from build123d import *

# Parameters (mm, degrees)
SKETCH1_W           = 127
SKETCH1_H           = 508
BOSS_EXTRUDE1_DEPTH = 95.25
SKETCH2_W           = 88.9
SKETCH2_H           = 469.9
CUT_EXTRUDE2_DEPTH  = 88.9
CUT_EXTRUDE3_DEPTH  = 128
SKETCH4_W           = 127
SKETCH4_H           = 19.05
CUT_EXTRUDE4_DEPTH  = 50.8


with BuildPart() as part:
    # Sketch1 → Boss-Extrude1 (new body)
    with BuildSketch(Plane(origin=(0, 0, 0), x_dir=(1, 0, 0), z_dir=(0, 1, 0))):
        Rectangle(SKETCH1_W, SKETCH1_H)
    extrude(amount=BOSS_EXTRUDE1_DEPTH)

    # Sketch2 → Cut-Extrude2 (cut)
    with BuildSketch(Plane(origin=(0, 95.25, 0), x_dir=(1, 0, 0), z_dir=(0, 1, 0))):
        Rectangle(SKETCH2_W, SKETCH2_H)
    extrude(amount=-CUT_EXTRUDE2_DEPTH, mode=Mode.SUBTRACT)

    # Sketch3 → Cut-Extrude3 (cut, through all)
    with BuildSketch(Plane(origin=(63.5, 0, 0), x_dir=(0, 0, -1), z_dir=(1, 0, 0))):
        with BuildLine():
            Line((203.2, 38.1), (-215.9, 38.1))
            ThreePointArc((-215.9, 38.1), (-228.6, 50.8), (-215.9, 63.5))
            Line((-215.9, 63.5), (203.2, 63.5))
            ThreePointArc((203.2, 63.5), (215.9, 50.8), (203.2, 38.1))
        make_face()
    extrude(amount=-CUT_EXTRUDE3_DEPTH, mode=Mode.SUBTRACT)

    # Sketch4 → Cut-Extrude4 (cut)
    with BuildSketch(Plane.XY.offset(254)):
        with Locations((0, 9.525)):
            Rectangle(SKETCH4_W, SKETCH4_H)
    extrude(amount=-CUT_EXTRUDE4_DEPTH, mode=Mode.SUBTRACT)


solid = part.part
Design review of the part built by this model. Coordinates are the model's own, in mm. A direction names the side the tool comes from. Round coordinates to 2 decimals unless told otherwise and drop trailing zeros. Loops run counter-clockwise (first coordinate to the right, second up) from the corner with the lowest first, then second, coordinate; pieces in that order, holes last. Notation, with made-up numbers: (29.5, 73) - (73.5, 73) arc R28 ccw to (73.5, 97) - close; hole circle Ø4 at (84.5, 46.25). An arc over 180 degrees is marked (long way). One line per item, written item: value. Start each with the question number.
1) Consider section A-A on x = 37.5. Give the boundary of the cut face in (y, z).
2) Consider section C-C on y = 11. Give the boundary of the cut face in (x, z).
3) To check wall thickness, follow L1, parallel to X at y = 82.5, z = 146.5; L2, parallel to Z at x = 3, y = 80; L3, parallel to Y at x = -24.5, z = 47. State the ranges of each line that lie inside material, in increasing order. Write a range as from..to.
4) For faces 5 (the flat face through (-1, 58, 234.95)), 6 (the flat face through (-1, 51, -234.95)), 7 (the flat face through (54, 63.5, 9)), list the 3-axis set-ups (+Z, -Z, +X, -X, +Y, -Y) from which the entire face can be reached by the end or side of a thin tool; tool diameter is ignored.
5) Insertion check: pin 1 Ø1.5 at (x, z) = (-3.5, 48) entering from +Y; pin 2 Ø15 at (x, z) = (-5.5, 230) entering from -Y. Each pin has a flat end and moves straight along its axis. Give the tip position at first contact, or say it passes through.
6) Consider section D-D on y = 33. Give the boundary of the cut face in (x, z).
7) Consider section B-B on z = 24. Give the boundary of the cut face in (x, y), then the cut area to 3 significant figures.
8) Draft analysis for pull direction Z (two halves, no side actions). For faces 1 (the cylindrical face through (-53.842, 50.521, 228.597)), 2 (the flat face through (-1, 5, 203.2)), 3 (the flat face through (-1, 47, -254)), 4 (the flat face through (-47, 95.25, 18)), state which applies: +Z half, -Z half, draft (parallel to the pull), parting line (faces both ways), or undercut.
Reported:
1. outline: (0, -254) - (95.25, -254) - (95.25, -234.95) - (6.35, -234.95) - (6.35, 203.2) - (0, 203.2) - close; (19.05, 234.95) - (95.25, 234.95) - (95.25, 254) - (19.05, 254) - close
2. outline: (-63.5, -254) - (63.5, -254) - (63.5, 203.2) - (44.45, 203.2) - (44.45, -234.95) - (-44.45, -234.95) - (-44.45, 203.2) - (-63.5, 203.2) - close
3. L1: x = -63.5..-44.45, 44.45..63.5
3. L2: z = -254..-234.95, 234.95..254
3. L3: y = 0..6.35
4. face 5: +Y, -Y
4. face 6: +Y
4. face 7: +X, -X
5. pin 1: stops at y = 6.35
5. pin 2: stops at y = 19.05
6. outline: (-63.5, -254) - (63.5, -254) - (63.5, 254) - (-63.5, 254) - close; hole (-44.45, -234.95) - (44.45, -234.95) - (44.45, 234.95) - (-44.45, 234.95) - close
7. outline: (-63.5, 0) - (63.5, 0) - (63.5, 38.1) - (44.45, 38.1) - (44.45, 6.35) - (-44.45, 6.35) - (-44.45, 38.1) - (-63.5, 38.1) - close; (-63.5, 63.5) - (-44.45, 63.5) - (-44.45, 95.25) - (-63.5, 95.25) - close; (44.45, 63.5) - (63.5, 63.5) - (63.5, 95.25) - (44.45, 95.25) - close
7. area: 3,230 mm^2
8. face 1: undercut
8. face 2: +Z half
8. face 3: -Z half
8. face 4: draft
